Model file for the job. Use its own axes, mm. A direction names the side the tool comes from. Coordinates: 2 decimals unless noted, no trailing zeros. Order: outer loops, then holes, each group sorted by start corner. A loop starts at its lowest first (then second) coordinate and runs counter-clockwise, first axis right, second up.
Autodesk Inventor part; units mm, degrees
ref_plane "YZ Plane" through (0, 0, 0) normal (1, 0, 0) x (0, 1, 0)
ref_plane "XZ Plane" through (0, 0, 0) normal (0, 1, 0) x (-1, 0, 0)
ref_plane "XY Plane" through (0, 0, 0) normal (0, 0, 1) x (1, 0, 0)
sketch "Sketch1" plane through (0, 0, 0) normal (0, 0, 1) x (1, 0, 0)
  line L0 (12.7, 25.4) -> (-12.7, 25.4)
  line L1 (-12.7, 25.4) -> (-12.7, -25.4)
  line L2 (-12.7, -25.4) -> (12.7, -25.4)
  line L3 (12.7, -25.4) -> (12.7, 25.4)
  line L4 (12.7, 25.4) -> (-12.7, -25.4) construction
  line L5 (-12.7, 25.4) -> (12.7, -25.4) construction
  line L6 (-11.684, 24.384) -> (11.684, 24.384)
  line L7 (11.684, 24.384) -> (11.684, -24.384)
  line L8 (11.684, -24.384) -> (-11.684, -24.384)
  line L9 (-11.684, -24.384) -> (-11.684, 24.384)
  point P0 (0, 0)
  dimension "d0" = 1.016
  dimension "d1" = 50.8
  dimension "d2" = 25.4
extrude "Tube Length" add sketch "Sketch1" along normal mid plane 609.6
sketch "Sketch2" plane through (-12.7, 25.4, 304.8) normal (0, 1, 0) x (1, 0, 0)
  line L0 (0, 0) -> (0, 609.6)
  line L1 (25.4, 0) -> (0, 0)
  line L2 (25.4, 609.6) -> (25.4, 0)
  line L3 (0, 609.6) -> (25.4, 609.6)
  line L4 (25.4, 0) -> (0, 0)
  line L5 (12.7, 0) -> (12.7, 12.7) construction
  circle A0 centre (12.7, 12.7) radius 2.2479
  point P0 (12.7, 304.8)
  dimension "d5" = 12.7
  dimension "d6" = 4.4958
extrude "Top Hole" cut sketch "Sketch2" against normal through all contours A0
sketch "Sketch3" plane through (0, 0, 304.8) normal (0, 0, 1) x (1, 0, 0)
  line L0 (0, 0) -> (0, 25.4) construction
  line L1 (12.7, 25.4) -> (-12.7, 25.4)
  line L2 (-0.0508, 25.4) -> (0, 25.2984)
  line L3 (0.0508, 25.4) -> (0, 25.2984)
  line L4 (-12.7, 12.6492) -> (-12.5984, 12.7)
  line L5 (-12.7, 12.7508) -> (-12.5984, 12.7)
  line L6 (-12.7, -0.0508) -> (-12.5984, 0)
  line L7 (-12.7, 0.0508) -> (-12.5984, 0)
  line L8 (-12.7, -12.7508) -> (-12.5984, -12.7)
  line L9 (-12.7, -12.6492) -> (-12.5984, -12.7)
  line L10 (12.7, 0.0508) -> (12.5984, 0)
  line L11 (12.7, 12.6492) -> (12.5984, 12.7)
  line L12 (12.7, 12.7508) -> (12.5984, 12.7)
  line L13 (12.7, -0.0508) -> (12.5984, 0)
  line L14 (12.7, -12.6492) -> (12.5984, -12.7)
  line L15 (12.7, -12.7508) -> (12.5984, -12.7)
  line L16 (0.0508, -25.4) -> (0, -25.2984)
  line L17 (-0.0508, -25.4) -> (0, -25.2984)
  line L18 (-12.7, 25.4) -> (-12.7, -25.4)
  line L19 (12.7, -25.4) -> (12.7, 25.4)
  line L20 (-12.7, -25.4) -> (12.7, -25.4)
  point P0 (0, 12.7)
  point P1 (-12.7, 12.7)
  point P2 (-12.7, 0)
  point P3 (-12.7, -12.7)
  point P4 (12.7, 12.7)
  point P5 (12.7, 0)
  point P6 (12.7, -12.7)
  point P7 (0, -25.4)
  dimension "d12" = 0.1016
  dimension "d13" = 0.1016
  dimension "d16" = 90
  dimension "d20" = 12.7
  dimension "d27" = 360
pattern_linear "Rectangular Pattern1" count 24 spacing 25.4 along (0, 0, -1) of "Top Hole"
equation "\"d13\" = d12"
properties part number "Elevator Base Tube" material "Aluminum 6061"
Q1. Drop a flat-ended pin along its axis: P1, Ø2.5, axis at x = 0, z = -12.7, coming from the -Y side. Give the stop position or say it passes through.
Established:
P1: passes through
Q2. Probe line 1 (Y direction, x = 8, z = -137); line 2 (X direction, y = 20.5, z = -80); line 3 (X direction, y = -24.6, z = 38.1). List the from-to ranges inside material, lowest first.
Established:
line 1: y = -25.4 to -24.38, 24.38 to 25.4
line 2: x = -12.7 to -11.68, 11.68 to 12.7
line 3: x = -12.7 to -2.25, 2.25 to 12.7
Q3. Cut at A-A, the plane x = -7.25. List the corners of the cut face in (y, z).
Established:
outline: (-25.4, -304.8) - (-24.38, -304.8) - (-24.38, 304.8) - (-25.4, 304.8) - close; (24.38, -304.8) - (25.4, -304.8) - (25.4, 304.8) - (24.38, 304.8) - close
Q4. Mould opens along X. For faces 1 (the face through (0, -24.384, -4)), 2 (the face through (0, 25.4, -4)), 3 (the face through (12.7, 0, -4)) say: pulls with the +X half, pulls with the -X half, needs draft (parallel to the pull), parting line crosses it, or undercut.
Established:
face 1: undercut
face 2: needs draft
face 3: pulls with the +X half
Q5. Which spindle directions (+Z, -Z, +X, -X, +Y, -Y) get a long thin tool onto all of the face, cutting with end or side? Do faces 4 (the face through (-11.684, 0, -4)), 5 (the face through (12, 8, 304.8)). Say none if no direction does.
Established:
face 4: +Z, -Z
face 5: +Z, +X, -X, +Y, -Y
Q6. Cut at C-C, the plane y = 16. List the corners of the cut face in (x, z).
Established:
outline: (-12.7, -304.8) - (-11.68, -304.8) - (-11.68, 304.8) - (-12.7, 304.8) - close; (11.68, -304.8) - (12.7, -304.8) - (12.7, 304.8) - (11.68, 304.8) - close
Q7. Cut at B-B, the plane z = -99. List the corners of the cut face in (x, y), plus the area to 3 significant figures.
Established:
outline: (-12.7, -25.4) - (12.7, -25.4) - (12.7, 25.4) - (-12.7, 25.4) - close; hole (-11.68, -24.38) - (11.68, -24.38) - (11.68, 24.38) - (-11.68, 24.38) - close
area: 151 mm2
